Check sheet for the modelled part. Datum: model origin and axes. Units: mm. Give positions to 0.01 mm unless a question says otherwise; leave off trailing zeros. Loops run counter-clockwise (first coordinate to the right, second up) from the corner with the lowest first, then second, coordinate; pieces in that order, holes last. Notation, with made-up numbers: (-38, 24) - (-24, 24) arc R21 cw to (-24, 57) - close; hole circle Ø5 at (-13, 66.25). An arc over 180 degrees is marked (long way). Answer in a Markdown table with one row per item. Add a question column.
(1) Sectioned sample at B-B on y = 3.25. Enter the section's corners in (x, z).
(2) Sectioned sample at C-C on x = 19.05. Enter the section's corners in (y, z), then the cut area to 3 significant figures.
(3) Thickness scan on L1, parallel to Z at x = 21.5, y = 1.75; L2, parallel to X at y = 4.25, z = -12.7; L3, parallel to Z at x = 24.5, y = 4.5. Record the ranges inside material, lowest first.
(4) Sectioned sample at D-D on z = -77. Enter the section's corners in (x, y), then the cut area to 3 significant figures.
(5) Sectioned sample at A-A on z = -50.8. Enter the section's corners in (x, y).
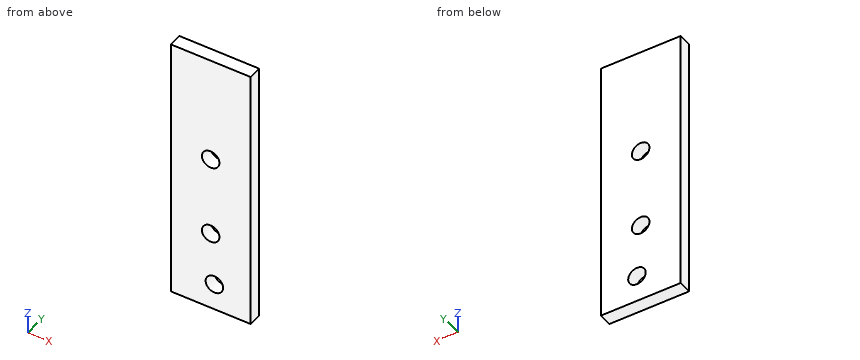
from build123d import *

# Parameters (mm, degrees)
SKETCH1_W           = 38.1
SKETCH1_H           = 88.9
SKETCH1_R           = 4.191
BOSS_EXTRUDE1_DEPTH = 6.35
SKETCH3_W           = 38.1
SKETCH3_H           = 6.35
BOSS_EXTRUDE2_DEPTH = 38.1


with BuildPart() as part:
    # Sketch1 → Boss-Extrude1 (new body)
    with BuildSketch(Plane(origin=(0, 0, 0), x_dir=(1, 0, 0), z_dir=(0, 1, 0))):
        with Locations((19.05, 44.45)):
            Rectangle(SKETCH1_W, SKETCH1_H)
        with Locations(Location((19.05, 12.7, 0), (0, 0, 270))):
            Circle(SKETCH1_R, mode=Mode.SUBTRACT)
        with Locations(Location((19.05, 50.8, 0), (0, 0, 270))):
            Circle(SKETCH1_R, mode=Mode.SUBTRACT)
        with Locations(Location((20.821814433, 76.138126877, 0), (0, 0, 270))):
            Circle(SKETCH1_R, mode=Mode.SUBTRACT)
    extrude(amount=BOSS_EXTRUDE1_DEPTH)

    # Sketch3 → Boss-Extrude2 (add)
    with BuildSketch(Plane.XY):
        with Locations((19.05, 3.175)):
            Rectangle(SKETCH3_W, SKETCH3_H)
    extrude(amount=BOSS_EXTRUDE2_DEPTH)


solid = part.part
Reply:
| question | item | result |
|---|---|---|
| 1 | outline | (0, -88.9) - (38.1, -88.9) - (38.1, 38.1) - (0, 38.1) - close; hole circle Ø8.38 at (19.05, -50.8); hole circle Ø8.38 at (19.05, -12.7); hole circle Ø8.38 at (20.82, -76.14) |
| 2 | outline | (0, -88.9) - (6.35, -88.9) - (6.35, -79.94) - (0, -79.94) - close; (0, -72.34) - (6.35, -72.34) - (6.35, -54.99) - (0, -54.99) - close; (0, -46.61) - (6.35, -46.61) - (6.35, -16.89) - (0, -16.89) - close; (0, -8.51) - (6.35, -8.51) - (6.35, 38.1) - (0, 38.1) - close |
| 2 | area | 652 mm^2 |
| 3 | L1 | -88.9 to -80.27, -72 to -54.2, -47.4 to -16.1, -9.3 to 38.1 |
| 3 | L2 | 0 to 14.86, 23.24 to 38.1 |
| 3 | L3 | -88.9 to -78.15, -74.13 to 38.1 |
| 4 | outline | (0, 0) - (16.72, 0) - (16.72, 6.35) - (0, 6.35) - close; (24.92, 0) - (38.1, 0) - (38.1, 6.35) - (24.92, 6.35) - close |
| 4 | area | 190 mm^2 |
| 5 | outline | (0, 0) - (14.86, 0) - (14.86, 6.35) - (0, 6.35) - close; (23.24, 0) - (38.1, 0) - (38.1, 6.35) - (23.24, 6.35) - close |
